```python
from build123d import *

# Parameters (mm, degrees)
SKETCH_1_R          = 41
SKETCH_1_R_2        = 4
SKETCH_1_R_3        = 2
EXTRUDE_1_DEPTH     = 15
CUT_EXTRUDE_START   = -13
SKETCH_3_R          = 41
SKETCH_3_R_2        = 37.815
CUT_EXTRUDE_1_DEPTH = 11


with BuildPart() as part:
    # 草图1 → 凸台-拉伸1 (new body)
    with BuildSketch(Plane.XY):
        Circle(SKETCH_1_R)
        Circle(SKETCH_1_R_2, mode=Mode.SUBTRACT)
        with Locations((-17.5, 0)):
            Circle(SKETCH_1_R_3, mode=Mode.SUBTRACT)
        with Locations((0, 17.5)):
            Circle(SKETCH_1_R_3, mode=Mode.SUBTRACT)
        with Locations((17.5, 0)):
            Circle(SKETCH_1_R_3, mode=Mode.SUBTRACT)
        with Locations((0, -17.5)):
            Circle(SKETCH_1_R_3, mode=Mode.SUBTRACT)
    extrude(amount=EXTRUDE_1_DEPTH)

    # 草图3 → 切除-拉伸1 (cut)
    with BuildSketch(Plane.XY.offset(15).offset(CUT_EXTRUDE_START)):
        Circle(SKETCH_3_R)
        Circle(SKETCH_3_R_2, mode=Mode.SUBTRACT)
    extrude(amount=CUT_EXTRUDE_1_DEPTH, mode=Mode.SUBTRACT)


solid = part.part
```
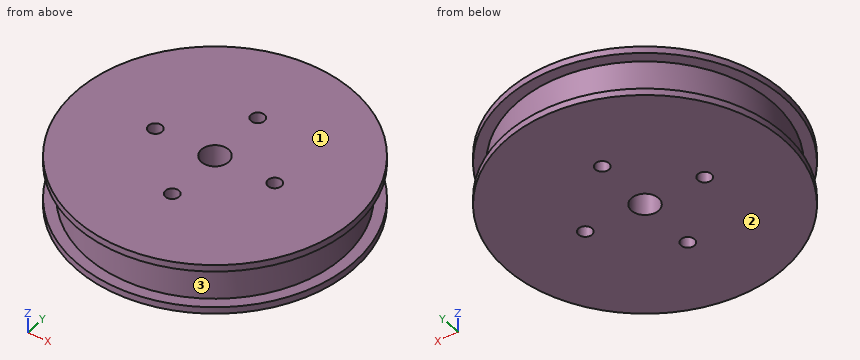
Work out the finished part from the listing and answer in its coordinate system (mm). Face numbers are marked on the shaded views. Round coordinates to 2 decimals unless told otherwise and drop trailing zeros. Write each loop counter-clockwise with the first axis right and the second up, starting at its lowest first coordinate (ties: lowest second). Pieces come first, ordered by that corner, then holes.
1) Determine the mould class of the marked faces 1, 2 and 3 for opening direction Z: pulls with the +Z half, pulls with the -Z half, needs draft (parallel to the pull), parting line crosses it, or undercut.
2) A cutting plane is placed at A-A on x = 0. Determine the outline of the cut face in (y, z) (3 decimals), and give its area (3 significant figures).
3) A cutting plane is placed at D-D on y = 17.5. Determine the outline of the cut face in (x, z), and give its area (3 significant figures).
4) A cutting plane is placed at B-B on z = 12. Determine the outline of the cut face in (x, y) (3 decimals), and give its area (3 significant figures).
5) Consider probe 1 along Y at (x, z) = (0, 6) (3 decimals); probe 2 along Z at (x, y) = (22.5, -31); probe 3 along X at (y, z) = (16, 14.75). Determine where each line is inside the solid, lowest interval first.
6) Flat-ended cylindrical pins translate along their axes: P1, Ø1, axis at y = -17, z = 5, coming from the +X side; P2, Ø1.5, axis at y = -27, z = 7, coming from the +X side; P3, Ø3, axis at y = 15, z = 5.5, coming from the -X side. Find the tip coordinate at first contact, or state that the pin passes through.
Entries:
1. face 1: pulls with the +Z half
1. face 2: pulls with the -Z half
1. face 3: undercut
2. outline: (-41, 0) - (-19.5, 0) - (-19.5, 15) - (-41, 15) - (-41, 13) - (-37.815, 13) - (-37.815, 2) - (-41, 2) - close; (-15.5, 0) - (-4, 0) - (-4, 15) - (-15.5, 15) - close; (4, 0) - (15.5, 0) - (15.5, 15) - (4, 15) - close; (19.5, 0) - (41, 0) - (41, 2) - (37.815, 2) - (37.815, 13) - (41, 13) - (41, 15) - (19.5, 15) - close
2. area: 920 mm2
3. outline: (-37.08, 0) - (-2, 0) - (-2, 15) - (-37.08, 15) - (-37.08, 13) - (-33.52, 13) - (-33.52, 2) - (-37.08, 2) - close; (2, 0) - (37.08, 0) - (37.08, 2) - (33.52, 2) - (33.52, 13) - (37.08, 13) - (37.08, 15) - (2, 15) - close
3. area: 974 mm2
4. outline: circle Ø75.63 at (0, 0); hole circle Ø4 at (-17.5, 0); hole circle Ø8 at (0, 0); hole circle Ø4 at (0, -17.5); hole circle Ø4 at (0, 17.5); hole circle Ø4 at (17.5, 0)
4. area: 4,390 mm2
5. probe 1: y = -37.815 to -19.5, -15.5 to -4, 4 to 15.5, 19.5 to 37.815
5. probe 2: z = 0 to 2, 13 to 15
5. probe 3: x = -37.75 to -1.32, 1.32 to 37.75
6. P1: stops at x = 34.03
6. P2: stops at x = 27.22
6. P3: stops at x = -35.32
